from build123d import *

# Parameters (mm, degrees)
SKETCH_W     = 19.8
SKETCH_H     = 8.4
PAD_DEPTH    = 14.12
SKETCH001_W  = 29.65
SKETCH001_H  = 8.4
PAD001_DEPTH = 1
SKETCH002_R  = 1
POCKET_DEPTH = 15.121
SKETCH003_W  = 19.8
SKETCH003_H  = 8.4
PAD002_DEPTH = 8.1


with BuildPart() as part:
    # Sketch → Pad (new body)
    with BuildSketch(Plane.XY):
        with Locations((9.9, 4.2)):
            Rectangle(SKETCH_W, SKETCH_H)
    extrude(amount=PAD_DEPTH)

    # Sketch001 → Pad001 (new body)
    with BuildSketch(Plane.XY.offset(14.12)):
        with Locations((9.9, 4.2)):
            Rectangle(SKETCH001_W, SKETCH001_H)
    extrude(amount=PAD001_DEPTH)

    # Sketch002 → Pocket (cut, through all)
    with BuildSketch(Plane.XY.offset(15.12)):
        with Locations((-1.6, 4.2)):
            Circle(SKETCH002_R)
        with Locations((21.4, 4.2)):
            Circle(SKETCH002_R)
    extrude(amount=-POCKET_DEPTH, mode=Mode.SUBTRACT)

    # Sketch003 → Pad002 (new body)
    with BuildSketch(Plane.XY.offset(15.12)):
        with Locations((9.9, 4.2)):
            Rectangle(SKETCH003_W, SKETCH003_H)
    extrude(amount=PAD002_DEPTH)


solid = part.part
Geometry: final body of the model. Coordinates: model frame, mm. A direction names the side the tool comes from. Round coordinates to 2 decimals unless told otherwise and drop trailing zeros. Loops run counter-clockwise (first coordinate to the right, second up) from the corner with the lowest first, then second, coordinate; pieces in that order, holes last.
Q1. Pin query (flat end, axial travel): P1, Ø1.5, axis at x = 15.5, z = 18, coming from the -Y side; P2, Ø1.5, axis at y = 7, z = 11, coming from the -X side; P3, Ø2.5, axis at x = 21.4, y = 4.2, coming from the +Z side; P4, Ø2.5, axis at x = -1.6, y = 4.2, coming from the -Z side. Return the tip coordinate at first contact, or that it passes through.
Q2. Section B-B on x = -1.6. Return loops of the section in (y, z), plus the area to 3 significant figures.
Q3. Section D-D on x = 22. Return loops of the section in (y, z).
Q4. Access query for faces 1 (the flat face through (13, 8.4, 11)), 2 (the flat face through (0, 4, 19)), 3 (the flat face through (23, 4, 15.12)), 4 (the flat face through (23, 4, 14.12)), 5 (the flat face through (-3, 4, 14.12)). Directions: +Z, -Z, +X, -X, +Y, -Y. A direction counts if a zero-diameter tool reaches every point of the face in a straight line with its end or side. Return the directions, or none.
Q5. Section C-C on y = 6.5. Return loops of the section in (x, z) (3 decimals).
Q6. Section A-A on y = 4.2. Return loops of the section in (x, z) (3 decimals), plus the area to 3 significant figures.
Q7. Material intervals for L1, parallel to Y at x = -1.6, z = 14.75; L2, parallel to Z at x = -0.5, y = 5.75; L3, parallel to X at y = 1, z = 5.25, sorted ascending.
Q8. Pull-direction query (Y, two-part tool) for faces 6 (the flat face through (13, 0, 11)), 7 (the cylindrical face through (22.324, 3.817, 14.627)), 8 (the flat face through (0, 4, 7)), 9 (the cylindrical face through (-1.14, 3.31, 14.63)); classes: released by +Y, released by -Y, zero draft, split by the parting line, or undercut.
Evaluation:
1. P1: stops at y = 0
1. P2: stops at x = 0
1. P3: stops at z = 15.12
1. P4: stops at z = 14.12
2. outline: (0, 14.12) - (3.2, 14.12) - (3.2, 15.12) - (0, 15.12) - close; (5.2, 14.12) - (8.4, 14.12) - (8.4, 15.12) - (5.2, 15.12) - close
2. area: 6.40 mm2
3. outline: (0, 14.12) - (3.4, 14.12) - (3.4, 15.12) - (0, 15.12) - close; (5, 14.12) - (8.4, 14.12) - (8.4, 15.12) - (5, 15.12) - close
4. face 1: +Z, -Z, +X, -X, +Y
4. face 2: +Z, -X, +Y, -Y
4. face 3: +Z, +X, +Y, -Y
4. face 4: -Z, +X, +Y, -Y
4. face 5: -Z, -X, +Y, -Y
5. outline: (-4.925, 14.12) - (0, 14.12) - (0, 0) - (19.8, 0) - (19.8, 14.12) - (24.725, 14.12) - (24.725, 15.12) - (19.8, 15.12) - (19.8, 23.22) - (0, 23.22) - (0, 15.12) - (-4.925, 15.12) - close
6. outline: (-4.925, 14.12) - (-2.6, 14.12) - (-2.6, 15.12) - (-4.925, 15.12) - close; (-0.6, 14.12) - (0, 14.12) - (0, 0) - (19.8, 0) - (19.8, 14.12) - (20.4, 14.12) - (20.4, 15.12) - (19.8, 15.12) - (19.8, 23.22) - (0, 23.22) - (0, 15.12) - (-0.6, 15.12) - close; (22.4, 14.12) - (24.725, 14.12) - (24.725, 15.12) - (22.4, 15.12) - close
6. area: 466 mm2
7. L1: y = 0 to 3.2, 5.2 to 8.4
7. L2: z = 14.12 to 15.12
7. L3: x = 0 to 19.8
8. face 6: released by -Y
8. face 7: undercut
8. face 8: zero draft
8. face 9: undercut
